```python
from build123d import *

# Parameters (mm, degrees)
F0_W     = 2.3323807579
F0_H     = 3
F1_DEPTH = 10
F2_R     = 3.5
F3_DEPTH = 4
F4_R     = 1.5
F5_R     = 1
F6_DEPTH = 25


with BuildPart() as f1:
    # F0 (on Top) → F1 (new body)
    with BuildSketch(Plane.XY):
        with BuildLine():
            Line((-1.166190379, -1.5), (-1.166190379, 1.5))
            ThreePointArc((-1.166190379, 1.5), (-1.9, 0), (-1.166190379, -1.5))
        make_face()
        with BuildLine():
            ThreePointArc((1.166190379, -1.5), (1.7067163971, -0.8349366084), (1.9, 0))
            ThreePointArc((1.9, 0), (1.7067163971, 0.8349366084), (1.166190379, 1.5))
            Line((1.166190379, 1.5), (1.166190379, -1.5))
        make_face()
        Rectangle(F0_W, F0_H)
    extrude(amount=F1_DEPTH)

    # F2 (on Top) → F3 (join)
    with BuildSketch(Plane.XY):
        Circle(F2_R)
    extrude(amount=F3_DEPTH)

    # F4
    f4_edges = [f1.edges().sort_by_distance(p)[0] for p in [
        (-1.9, 0, 4),
        (0, 1.5, 4),
        (0, -1.5, 4),
        (1.9, 0, 4),
    ]]
    fillet(f4_edges, radius=F4_R)

    # F5 (on face) → F6 (cut)
    with BuildSketch(Plane.XY.offset(10)):
        Circle(F5_R)
    extrude(amount=-F6_DEPTH, mode=Mode.SUBTRACT)


solid = f1.part
```
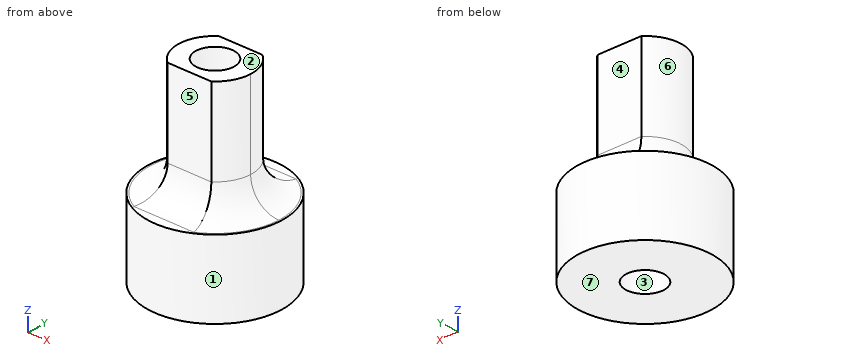
Model file for the job. Use its own axes, mm. Face numbers are marked on the shaded views. A direction names the side the tool comes from. Give positions to 0.01 mm unless a question says otherwise; leave off trailing zeros. Write each loop counter-clockwise with the first axis right and the second up, starting at its lowest first coordinate (ties: lowest second). Pieces come first, ordered by that corner, then holes. Notation, with made-up numbers: M 54.5,21 L 64.5,21 A37 ccw 64.5,60 Z; hole C 76.5,-38.75 d10. An arc over 180 degrees is marked long. Use a Markdown table: item, result.
1) Cut at C-C (z = 1.75). List the corners of the cut face in (x, y), and give its area (3 significant figures).
Responses:
| item | result |
|---|---|
| outline | C 0,0 d7; hole C 0,0 d2 |
| area | 35.3 mm2 |
2) Tool access for the marked faces 5, 6 and 7: list every direction of +Z, -Z, +X, -X, +Y, -Y with a clear straight run to the whole face (end or side of a thin tool).
Responses:
| item | result |
|---|---|
| face 5 | +Z, +X, -X, -Y |
| face 6 | +Z, -X |
| face 7 | -Z, +X, -X, +Y, -Y |
3) Drill centre lines: line 1 (Y direction, x = 0, z = 6); line 2 (Y direction, x = 0, z = 3.5); line 3 (X direction, y = -0.75, z = 3.5). Where is each one in solid material? Low to high. Write a range as from..to.
Responses:
| item | result |
|---|---|
| line 1 | y = -1.5..-1, 1..1.5 |
| line 2 | y = -3.5..-1, 1..3.5 |
| line 3 | x = -3.42..-0.66, 0.66..3.42 |
4) Pull direction Y, two halves, no side cores. Call the marked faces 1, 2, 3 and 4: +Y half, -Y half, draft (parallel to the pull), parting line (faces both ways), or undercut.
Responses:
| item | result |
|---|---|
| face 1 | parting line |
| face 2 | draft |
| face 3 | undercut |
| face 4 | +Y half |
5) Cut at B-B (z = 6). List the corners of the cut face in (x, y), and give its area (3 significant figures).
Responses:
| item | result |
|---|---|
| outline | M -1.17,-1.5 L 1.17,-1.5 A1.9 ccw 1.17,1.5 L -1.17,1.5 A1.9 ccw Z; hole C 0,0 d2 |
| area | 6.93 mm2 |
6) Cut at A-A (x = 0). List the corners of the cut face in (y, z), and give its area (3 significant figures).
Responses:
| item | result |
|---|---|
| outline | M -3.5,0 L -1,0 L -1,10 L -1.5,10 L -1.5,5.5 A1.5 cw -3,4 L -3.5,4 Z; M 1,0 L 3.5,0 L 3.5,4 L 3,4 A1.5 cw 1.5,5.5 L 1.5,10 L 1,10 Z |
| area | 27.0 mm2 |
7) Pin check, flat tips, straight feed: pin 1 (1.2 mm diameter, centred on x = 0.5, z = 7.5, fed in from +Y); pin 2 (4 mm diameter, centred on y = -1, z = 8.5, fed in from -X); pin 3 (1.5 mm diameter, centred on x = -1, y = 0, fed in from -Z); pin 4 (0.7 mm diameter, centred on x = -0.5, z = 9, fed in from -Y). Stop position of each tip, or through.
Responses:
| item | result |
|---|---|
| pin 1 | stops at y = 1.5 |
| pin 2 | stops at x = -1.9 |
| pin 3 | stops at z = 0 |
| pin 4 | stops at y = -1.5 |
